Model file for the job. Use its own axes, mm. A direction names the side the tool comes from. Round coordinates to 2 decimals unless told otherwise and drop trailing zeros. Order: outer loops, then holes, each group sorted by start corner. A loop starts at its lowest first (then second) coordinate and runs counter-clockwise, first axis right, second up. Notation, with made-up numbers: (-12, -32.5) - (16, -32.5) arc R18 cw to (16, -18.5) - close; hole circle Ø10 at (47, -24). An arc over 180 degrees is marked (long way). Put each result on its own line as item: value. Start each with the question number.
Item 1: Probe probe 1 along Y at (x, z) = (54, 2.8); probe 2 along Y at (x, z) = (25, 2.5); probe 3 along X at (y, z) = (45.5, 2). List the from-to ranges inside material, lowest first.
Item 2: Saw through at C-C on x = 11. List the corners of the cut face in (y, z).
Item 3: Pin check, flat tips, straight feed: pin 1 Ø2 at (x, y) = (13.5, 61) entering from +Z; pin 2 Ø6.5 at (x, y) = (5, 6.5) entering from +Z; pin 3 Ø3 at (y, z) = (33, 3) entering from +X; pin 4 Ø3.5 at (x, y) = (64, 5) entering from +Z. Stop position of each tip, or through.
Item 4: Saw through at A-A on z = 4.5. State how many separate pieces and enclosed holes the cut face has, plus the area to 3 significant figures.
Item 5: Mould opens along Y. For faces 5 (the face through (62, 6, 1.5)), 6 (the face through (54, 5, 1.5)) say: pulls with the +Y half, pulls with the -Y half, needs draft (parallel to the pull), parting line crosses it, or undercut.
Item 6: Which spindle directions (+Z, -Z, +X, -X, +Y, -Y) get a long thin tool onto all of the face, cutting with end or side? Do faces 1 (the face through (63.21, 12.32, 0.74)), 2 (the face through (-9.587, 84.989, 0.74)), 3 (the face through (29, 87, 4)), 4 (the face through (-3, 82, 1.5)). Say none if no direction does.
Item 7: Saw through at B-B on y = 50. List the corners of the cut face in (x, z), plus the area to 3 significant figures.
Item 8: Saw through at D-D on x = 54. List the corners of the cut face in (y, z), plus the area to 3 significant figures.
```python
from build123d import *

# Parameters (mm, degrees)
SKETCH_R        = 2
PAD_DEPTH       = 1.5
SKETCH001_W     = 59
SKETCH001_H     = 88
PAD001_DEPTH    = 5
SKETCH002_W     = 57
SKETCH002_H     = 86
POCKET_DEPTH    = 5
SKETCH003_W     = 13
SKETCH003_H     = 3
POCKET001_DEPTH = 1
SKETCH004_R     = 3
SKETCH004_R_2   = 1.5
PAD002_DEPTH    = 4


with BuildPart() as part:
    # Sketch → Pad (new body)
    with BuildSketch(Plane.XY):
        with BuildLine():
            Line((0, 0), (59, 0))
            Line((63.999982, 0), (59, 0))
            ThreePointArc((63.999982, 0), (68.619394, 3.086575), (67.535534, 8.535534))
            Line((59, 16), (67.535534, 8.535534))
            Line((59, 16), (59, 72))
            Line((59, 72), (67.535534, 79.464466))
            ThreePointArc((67.535534, 79.464466), (68.619394, 84.913425), (63.999983, 88))
            Line((59, 88), (63.999983, 88))
            Line((59, 88), (0, 88))
            Line((-4.999983, 88), (0, 88))
            ThreePointArc((-4.999983, 88), (-9.619394, 84.913425), (-8.535534, 79.464466))
            Line((-8.535534, 79.464466), (0, 72))
            Line((0, 72), (0, 16))
            Line((-8.535534, 8.535534), (0, 16))
            ThreePointArc((-8.535534, 8.535534), (-9.619398, 3.086583), (-5, 0))
            Line((0, 0), (-5, 0))
        make_face()
        with Locations((-5, 83)):
            Circle(SKETCH_R, mode=Mode.SUBTRACT)
        with Locations((64, 83)):
            Circle(SKETCH_R, mode=Mode.SUBTRACT)
        with Locations((-5, 5)):
            Circle(SKETCH_R, mode=Mode.SUBTRACT)
        with Locations((64, 5)):
            Circle(SKETCH_R, mode=Mode.SUBTRACT)
    extrude(amount=PAD_DEPTH)

    # Sketch001 → Pad001 (new body)
    with BuildSketch(Plane.XY.offset(1.5)):
        with Locations((29.5, 44)):
            Rectangle(SKETCH001_W, SKETCH001_H)
    extrude(amount=PAD001_DEPTH)

    # Sketch002 → Pocket (cut)
    with BuildSketch(Plane.XY.offset(6.5)):
        with Locations((29.5, 44)):
            Rectangle(SKETCH002_W, SKETCH002_H)
    extrude(amount=-POCKET_DEPTH, mode=Mode.SUBTRACT)

    # Sketch003 → Pocket001 (cut)
    with BuildSketch(Plane.XZ):
        with Locations((29.5, 5)):
            Rectangle(SKETCH003_W, SKETCH003_H)
    extrude(amount=-POCKET001_DEPTH, mode=Mode.SUBTRACT)

    # Sketch004 → Pad002 (new body)
    with BuildSketch(Plane.XY.offset(1.5)):
        with Locations((5, 63)):
            Circle(SKETCH004_R)
        with Locations((5, 63)):
            Circle(SKETCH004_R_2, mode=Mode.SUBTRACT)
        with Locations((54, 63)):
            Circle(SKETCH004_R)
        with Locations((54, 63)):
            Circle(SKETCH004_R_2, mode=Mode.SUBTRACT)
        with Locations((5, 5)):
            Circle(SKETCH004_R)
        with Locations((5, 5)):
            Circle(SKETCH004_R_2, mode=Mode.SUBTRACT)
        with Locations((54, 5)):
            Circle(SKETCH004_R)
        with Locations((54, 5)):
            Circle(SKETCH004_R_2, mode=Mode.SUBTRACT)
    extrude(amount=PAD002_DEPTH)


solid = part.part
```
Results found:
1. probe 1: y = 0 to 1, 2 to 3.5, 6.5 to 8, 60 to 61.5, 64.5 to 66, 87 to 88
1. probe 2: y = 0 to 1, 87 to 88
1. probe 3: x = 0 to 1, 58 to 59
2. outline: (0, 0) - (88, 0) - (88, 6.5) - (87, 6.5) - (87, 1.5) - (1, 1.5) - (1, 6.5) - (0, 6.5) - close
3. pin 1: stops at z = 1.5
3. pin 2: stops at z = 5.5
3. pin 3: stops at x = 59
3. pin 4: passes through
4. separate pieces: 5
4. enclosed holes: 4
4. area: 362 mm²
5. face 5: needs draft
5. face 6: undercut
6. face 1: +Z, -Z, +X
6. face 2: +Z, -Z, -X
6. face 3: +Z
6. face 4: +Z, -X, +Y, -Y
7. outline: (0, 0) - (59, 0) - (59, 6.5) - (58, 6.5) - (58, 1.5) - (1, 1.5) - (1, 6.5) - (0, 6.5) - close
7. area: 98.5 mm²
8. outline: (0, 0) - (88, 0) - (88, 6.5) - (87, 6.5) - (87, 1.5) - (66, 1.5) - (66, 5.5) - (64.5, 5.5) - (64.5, 1.5) - (61.5, 1.5) - (61.5, 5.5) - (60, 5.5) - (60, 1.5) - (8, 1.5) - (8, 5.5) - (6.5, 5.5) - (6.5, 1.5) - (3.5, 1.5) - (3.5, 5.5) - (2, 5.5) - (2, 1.5) - (1, 1.5) - (1, 6.5) - (0, 6.5) - close
8. area: 166 mm²
